from build123d import *

# Parameters (mm, degrees)
BOSS_EXTRUDE1_DEPTH      = 1.65
BOSS_EXTRUDE1_DEPTH_BACK = 1.65
CUT_EXTRUDE2_DEPTH       = 81
CUT_EXTRUDE2_DEPTH_BACK  = 103


with BuildPart() as part:
    # Sketch1 → Boss-Extrude1 (new, two sides: drawn at the far end of the back side and taken through both)
    with BuildSketch(Plane.XY.offset(-BOSS_EXTRUDE1_DEPTH_BACK)):
        with BuildLine():
            Line((-6.5, 0), (-15.242640687, 8))
            ThreePointArc((-15.242640687, 8), (-12.859499425, 16.676124215), (-5.5, 11.5))
            Line((-5.5, 11.5), (-5.5, 9))
            ThreePointArc((-5.5, 9), (-5.207106781, 8.292893219), (-4.5, 8))
            Line((-4.5, 8), (4.5, 8))
            ThreePointArc((4.5, 8), (5.207106781, 8.292893219), (5.5, 9))
            Line((5.5, 9), (5.5, 11.5))
            ThreePointArc((5.5, 11.5), (12.859499425, 16.676124215), (15.242640687, 8))
            Line((15.242640687, 8), (6.5, 0))
            Line((6.5, 0), (-6.5, 0))
        make_face()
    extrude(amount=BOSS_EXTRUDE1_DEPTH + BOSS_EXTRUDE1_DEPTH_BACK)

    # Sketch6 → Cut-Extrude2 (cut, two sides: drawn at the far end of the back side and taken through both)
    with BuildSketch(Plane(origin=(0, 0, 0), x_dir=(0, 0, -1), z_dir=(1, 0, 0)).offset(-CUT_EXTRUDE2_DEPTH_BACK)):
        Polygon((-3, 0), (-1.65, 0), (-1.15, 17), (-3, 17), align=None)
        Polygon((1.15, 17), (3, 17), (3, 0), (1.65, 0), align=None)
    extrude(amount=CUT_EXTRUDE2_DEPTH + CUT_EXTRUDE2_DEPTH_BACK, mode=Mode.SUBTRACT)

    # Sketch2 → Revolve1 (revolve)
    with BuildSketch(Plane(origin=(0, 0, 0), x_dir=(0, 0, -1), z_dir=(1, 0, 0))):
        with BuildLine():
            Line((0, 0), (-6.5, 0))
            Line((-6.5, 0), (-5.5, 7))
            ThreePointArc((-5.5, 7), (-5.207106781, 7.707106781), (-4.5, 8))
            Line((-4.5, 8), (0, 8))
            Line((0, 8), (0, 0))
        make_face()
    revolve(axis=Axis((0, 0, 0), (0, 1, 0)))

    # Sketch7 → Revolve2 (revolve)
    with BuildSketch(Plane(origin=(0, 0, 0), x_dir=(0, 0, -1), z_dir=(1, 0, 0))):
        Polygon((0, -25), (-2.9, -25), (-3, -24.9), (-3, 0), (0, 0), align=None)
    revolve(axis=Axis((0, 0, 0), (0, -1, 0)))


solid = part.part
The listing builds one solid part. Answer for the finished solid, in the listing's coordinates (mm). A direction names the side the tool comes from. Give positions to 0.01 mm unless a question says otherwise; leave off trailing zeros. Write each loop counter-clockwise with the first axis right and the second up, starting at its lowest first coordinate (ties: lowest second). Pieces come first, ordered by that corner, then holes. Notation, with made-up numbers: (55.25, -36) - (105.25, -36) arc R17 ccw to (105.25, -23) - close; hole circle Ø6 at (45.25, 74). An arc over 180 degrees is marked (long way). One line per question, with ' | ' between items. Start each with the question number.
1. Given P1, Ø3, axis at x = -7, z = 3, coming from the -Y side; P2, Ø4.5, axis at x = -1.5, z = -1, coming from the +Y side; P3, Ø1, axis at y = -14, z = -4.5, coming from the -X side; P4, Ø5, axis at y = -12.5, z = 2.5, coming from the +X side, each flat-ended and moving along its own axis, determine where each tip first touches the part or whether it passes through.
2. Section C-C, the plane y = 5 is taken. Determine the outline of the cut face in (x, z), then the cut area to 3 significant figures.
3. Section A-A, the plane y = 10.5 is taken. Determine the outline of the cut face in (x, z).
4. Section B-B, the plane z = 0 is taken. Determine the outline of the cut face in (x, y), then the cut area to 3 significant figures.
5. Straight lines are drawn through the part: line 1 (X direction, y = -16.5, z = -0.25); line 2 (Z direction, x = -9.5, y = 5); line 3 (Y direction, x = 1, z = -3). For each, find the intervals that lie inside material, in ascending order.
6. Determine the mould class of faces 4 (the face through (0, 8, 0)), 5 (the face through (10.933, 4.056, -0.023)), 6 (the face through (-10.81, 3.944, -0.023)) for opening direction X: +X half, -X half, draft (parallel to the pull), parting line (faces both ways), or undercut.
7. Section D-D, the plane x = -11 is taken. Determine the outline of the cut face in (y, z), then the cut area to 3 significant figures.
8. For faces 1 (the face through (0, -12, -3)), 2 (the face through (0, -25, 0)), 3 (the face through (-5.215, 8.301, -0.02)), determine the directions among +Z, -Z, +X, -X, +Y, -Y from which every point of the face is accessible in a straight line to the end or side of a thin tool.
Result:
1) P1: stops at y = 0 | P2: stops at y = 8 | P3: passes through | P4: stops at x = 3
2) outline: (-11.96, -1.5) - (-5.59, -1.5) arc R5.79 ccw to (5.59, -1.5) - (11.96, -1.5) - (11.96, 1.5) - (5.59, 1.5) arc R5.79 ccw to (-5.59, 1.5) - (-11.96, 1.5) - close | area: 143 mm2
3) outline: (-16.41, -1.34) - (-5.5, -1.34) - (-5.5, 1.34) - (-16.41, 1.34) - close; (5.5, -1.34) - (16.41, -1.34) - (16.41, 1.34) - (5.5, 1.34) - close
4) outline: (-15.24, 8) - (-6.5, 0) - (-3, 0) - (-3, -24.9) - (-2.9, -25) - (2.9, -25) - (3, -24.9) - (3, 0) - (6.5, 0) - (15.24, 8) arc R5.5 ccw (long way) to (5.5, 11.5) - (5.5, 9) arc R1 cw to (4.5, 8) - (-4.5, 8) arc R1 cw to (-5.5, 9) - (-5.5, 11.5) arc R5.5 ccw (long way) to start | area: 494 mm2
5) line 1: x = -2.99 to 2.99 | line 2: z = -1.5 to 1.5 | line 3: y = 0 to 8
6) face 4: undercut | face 5: +X half | face 6: -X half
7) outline: (4.12, -1.53) - (17, -1.15) - (17, 1.15) - (4.12, 1.53) - close | area: 34.5 mm2
8) face 1: -Y | face 2: +Z, -Z, +X, -X, -Y | face 3: +Z, -Z, +Y
